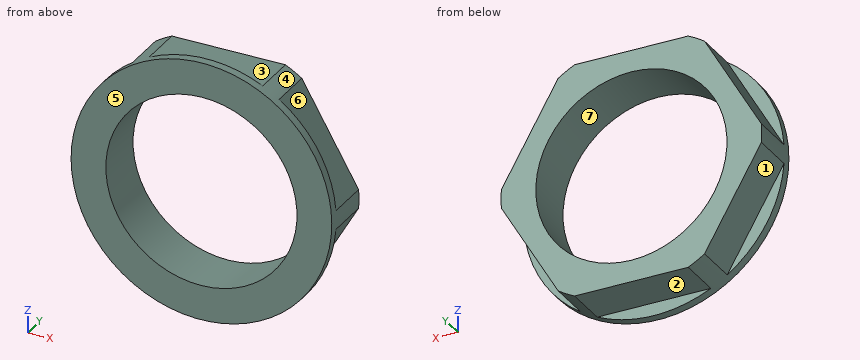
from build123d import *

# Parameters (mm, degrees)
SKIZZE1_R                       = 15
SKIZZE1_R_2                     = 11
AUFSATZ_LINEAR_AUSTRAGEN1_DEPTH = 1
SKIZZE2_R                       = 11
AUFSATZ_LINEAR_AUSTRAGEN2_DEPTH = 5
SKIZZE3_R                       = 15.588457268
SKIZZE3_R_2                     = 15
SCHNITT_LINEAR_AUSTRAGEN2_DEPTH = 23.449944321


with BuildPart() as part:
    # Skizze1 → Aufsatz-Linear austragen1 (new body)
    with BuildSketch(Plane(origin=(0, 0, 0), x_dir=(1, 0, 0), z_dir=(0, 1, 0))):
        with Locations(Location((0, 0, 0), (0, 0, 270))):
            Circle(SKIZZE1_R)
        with Locations(Location((0, 0, 0), (0, 0, 270))):
            Circle(SKIZZE1_R_2, mode=Mode.SUBTRACT)
    extrude(amount=AUFSATZ_LINEAR_AUSTRAGEN1_DEPTH)

    # Skizze2 → Aufsatz-Linear austragen2 (add)
    with BuildSketch(Plane(origin=(0, 1, 0), x_dir=(1, 0, 0), z_dir=(0, 1, 0))):
        Polygon((15.588457268, 0), (7.794228634, 13.5), (-7.794228634, 13.5), (-15.588457268, 0), (-7.794228634, -13.5), (7.794228634, -13.5), align=None)
        with Locations(Location((0, 0, 0), (0, 0, 270))):
            Circle(SKIZZE2_R, mode=Mode.SUBTRACT)
    extrude(amount=AUFSATZ_LINEAR_AUSTRAGEN2_DEPTH)

    # Skizze3 → Schnitt-Linear austragen2 (cut, through all)
    with BuildSketch(Plane(origin=(0, 6, 0), x_dir=(1, 0, 0), z_dir=(0, 1, 0))):
        Circle(SKIZZE3_R)
        with Locations(Location((0, 0, 0), (0, 0, 115.841932763))):
            Circle(SKIZZE3_R_2, mode=Mode.SUBTRACT)
    extrude(amount=-SCHNITT_LINEAR_AUSTRAGEN2_DEPTH, mode=Mode.SUBTRACT)


solid = part.part
Input: part model. Units: mm. Frame: model coordinates. Face numbers are marked on the shaded views. A direction names the side the tool comes from. Coordinates: 2 decimals unless noted, no trailing zeros. Loops run counter-clockwise (first coordinate to the right, second up) from the corner with the lowest first, then second, coordinate; pieces in that order, holes last. Notation, with made-up numbers: (24.5, 3.5) -> (32.5, 3.5) arc R23 cw to (32.5, 25.5) -> close; hole circle Ø6 at (80.5, 40). An arc over 180 degrees is marked (long way). Write each question's results on one line, items separated by ' | '. Start each with the question number.
Q1. Ray query, line 1 (X direction, y = 3.65, z = 0); line 2 (X direction, y = 3.4, z = 4.25); line 3 (Z direction, x = 9, y = 1.35). Return the intervals inside material, ascending. Write a range as from..to.
Q2. Reachability of the marked faces 1, 2 and 3 from +Z, -Z, +X, -X, +Y, -Y: full face, straight path, thin tool, end or side. Return the list, or none.
Q3. Section B-B, the plane x = 0. Return the cut outline in (y, z).
Q4. Section A-A, the plane z = 0. Return the cut outline in (x, y), plus the area to 3 significant figures.
Q5. Section D-D, the plane x = 7.5. Return the cut outline in (y, z), plus the area to 3 significant figures.
Q6. Pin query (flat end, axial travel): pin 1 (1.6 mm diameter, centred on x = -1.5, z = 14.5, fed in from +Y); pin 2 (1.5 mm diameter, centred on y = 1, z = 10, fed in from -X); pin 3 (3 mm diameter, centred on y = 3.5, z = -7, fed in from -X). Return the tip coordinate at first contact, or that it passes through.
Q7. Pull-direction query (X, two-part tool) for the marked faces 4, 5, 6 and 7; classes: released by +X, released by -X, zero draft, split by the parting line, or undercut.
Q8. Section C-C, the plane y = 2.7. Return the cut outline in (x, z), plus the area to 3 significant figures.
Found:
1) line 1: -15..-11, 11..15 | line 2: -13.13..-10.15, 10.15..13.13 | line 3: -11.41..-6.32, 6.32..11.41
2) face 1: -Z, -X, +Y | face 2: -Z, +X, -X, +Y | face 3: +Z, +X, -X, +Y
3) outline: (0, -15) -> (1, -15) -> (1, -13.5) -> (6, -13.5) -> (6, -11) -> (0, -11) -> close; (0, 11) -> (6, 11) -> (6, 13.5) -> (1, 13.5) -> (1, 15) -> (0, 15) -> close
4) outline: (-15, 0) -> (-11, 0) -> (-11, 6) -> (-15, 6) -> close; (11, 0) -> (15, 0) -> (15, 6) -> (11, 6) -> close | area: 48.0 mm2
5) outline: (0, -12.99) -> (6, -12.99) -> (6, -8.05) -> (0, -8.05) -> close; (0, 8.05) -> (6, 8.05) -> (6, 12.99) -> (0, 12.99) -> close | area: 59.3 mm2
6) pin 1: y = 1 | pin 2: x = -11.81 | pin 3: x = -12.41
7) face 4: split by the parting line | face 5: zero draft | face 6: released by +X | face 7: undercut
8) outline: (-14.96, -1.09) -> (-8.42, -12.41) arc R15 ccw to (-6.54, -13.5) -> (6.54, -13.5) arc R15 ccw to (8.42, -12.41) -> (14.96, -1.09) arc R15 ccw to (14.96, 1.09) -> (8.42, 12.41) arc R15 ccw to (6.54, 13.5) -> (-6.54, 13.5) arc R15 ccw to (-8.42, 12.41) -> (-14.96, 1.09) arc R15 ccw to start; hole circle Ø22 at (0, 0) | area: 247 mm2
